The listing builds one solid part. Answer for the finished solid, in the listing's coordinates (mm). A direction names the side the tool comes from. Coordinates: 2 decimals unless noted, no trailing zeros. Order: outer loops, then holes, each group sorted by start corner. A loop starts at its lowest first (then second) coordinate and runs counter-clockwise, first axis right, second up. Notation, with made-up numbers: (3, 57.5) -> (16, 57.5) arc R14 cw to (16, 84.5) -> close; hole circle Ø2 at (-37.75, -33.5). An arc over 180 degrees is marked (long way). Write item = value, one per line.
from build123d import *
from build123d.topology import SkipClean

# Parameters (mm, degrees)
SALIENTE_EXTRUIR1_DEPTH    = 2.4
CORTAR_EXTRUIR1_DEPTH      = 43.673293756
CORTAR_EXTRUIR1_DEPTH_BACK = 43.673293756
CROQUIS2_R                 = 1.5
CROQUIS3_R                 = 1.5
SALIENTE_EXTRUIR2_DEPTH    = 7.5
CORTAR_EXTRUIR2_DEPTH      = 3.1
REDONDEO1_R                = 2
REDONDEO2_R                = 1


with BuildPart() as part:
    # Croquis1 → Saliente-Extruir1 (new, symmetric)
    with BuildSketch(Plane(origin=(0, 0, 0), x_dir=(0, 0, -1), z_dir=(1, 0, 0))):
        with BuildLine():
            Line((-41.5, 3), (41.5, 3))
            ThreePointArc((41.5, 3), (42.207106781, 2.707106781), (42.5, 2))
            Line((42.5, 2), (42.5, -2))
            ThreePointArc((42.5, -2), (42.207106781, -2.707106781), (41.5, -3))
            Line((41.5, -3), (-41.5, -3))
            ThreePointArc((-41.5, -3), (-42.207106781, -2.707106781), (-42.5, -2))
            Line((-42.5, -2), (-42.5, 2))
            ThreePointArc((-42.5, 2), (-42.207106781, 2.707106781), (-41.5, 3))
        make_face()
    extrude(amount=SALIENTE_EXTRUIR1_DEPTH, both=True)

    # Croquis2 → Cortar-Extruir1 (cut, two sides: drawn at the far end of the back side and taken through both)
    with BuildSketch(Plane(origin=(0, 0, 0), x_dir=(0, 0, -1), z_dir=(1, 0, 0)).offset(-CORTAR_EXTRUIR1_DEPTH_BACK)):
        with Locations((-38.5, 0)):
            Circle(CROQUIS2_R)
        with Locations((33.5, 0)):
            Circle(CROQUIS2_R)
    extrude(amount=CORTAR_EXTRUIR1_DEPTH + CORTAR_EXTRUIR1_DEPTH_BACK, mode=Mode.SUBTRACT)

    # Croquis3 → Saliente-Extruir2 (add, symmetric)
    with SkipClean():  # the faces are left unmerged after this step: merging them gives an invalid solid
        with BuildSketch(Plane(origin=(0, 0, 0), x_dir=(0, 0, -1), z_dir=(1, 0, 0))):
            with BuildLine():
                Line((-42.5, 2), (-42.5, -2))
                ThreePointArc((-42.5, -2), (-42.207106781, -2.707106781), (-41.5, -3))
                Line((-41.5, -3), (-27.5, -3))
                Line((-27.5, -3), (-27.5, 3))
                Line((-27.5, 3), (-41.5, 3))
                ThreePointArc((-41.5, 3), (-42.207106781, 2.707106781), (-42.5, 2))
            make_face()
            with Locations((-38.5, 0)):
                Circle(CROQUIS3_R, mode=Mode.SUBTRACT)
        extrude(amount=SALIENTE_EXTRUIR2_DEPTH, both=True)
    add(part.part.scale(1), mode=Mode.REPLACE)  # the faces are merged on a copy

    # Croquis4 → Cortar-Extruir2 (cut, symmetric)
    with BuildSketch(Plane(origin=(0, 0, 0), x_dir=(0, 0, -1), z_dir=(1, 0, 0))):
        with BuildLine():
            Line((-41.5, 3), (-32.5, 3))
            Line((-32.5, 3), (-32.5, -3))
            Line((-32.5, -3), (-41.5, -3))
            ThreePointArc((-41.5, -3), (-42.207106781, -2.707106781), (-42.5, -2))
            Line((-42.5, -2), (-42.5, 2))
            ThreePointArc((-42.5, 2), (-42.207106781, 2.707106781), (-41.5, 3))
        make_face()
    extrude(amount=CORTAR_EXTRUIR2_DEPTH, both=True, mode=Mode.SUBTRACT)

    # Redondeo1
    redondeo1_edges = [part.edges().sort_by_distance(p)[0] for p in [
        (-2.4, 0, 27.5),
        (2.4, 0, 27.5),
        (-7.5, 0, 27.5),
        (7.5, 0, 27.5),
    ]]
    fillet(redondeo1_edges, radius=REDONDEO1_R)

    # Redondeo2
    redondeo2_edges = [part.edges().sort_by_distance(p)[0] for p in [
        (3.1, 0, 32.5),
        (-3.1, 0, 32.5),
    ]]
    fillet(redondeo2_edges, radius=REDONDEO2_R)


solid = part.part
Q1. Each of these flat-tipped pins is pushed along its axis until it touches: pin 1 Ø1.5 at (y, z) = (-0.5, 8) entering from +X; pin 2 Ø1 at (y, z) = (-1, -34) entering from -X; pin 3 Ø2 at (x, y) = (-1.5, 0.5) entering from +Z. Where does it stop, or does it pass through?
The answers:
pin_1 = 2.4
pin_2 = -2.4
pin_3 = 32.58
Q2. Section A-A, the plane x = 0.5 is taken. Give the vertices of the cut face in (y, z).
The answers:
outline = (-3, -41.5) arc R1 ccw to (-2, -42.5) -> (2, -42.5) arc R1 ccw to (3, -41.5) -> (3, 32.5) -> (-3, 32.5) -> close; hole circle Ø3 at (0, -33.5)
Q3. Section D-D, the plane z = 22 is taken. Give the vertices of the cut face in (x, y), plus the area to 3 significant figures.
The answers:
outline = (-2.4, -3) -> (2.4, -3) -> (2.4, 3) -> (-2.4, 3) -> close
area = 28.8 mm2
Q4. Section B-B, the plane y = 0 is taken. Give the number of separate pieces and of enclosed holes in the cut face, plus the area to 3 significant figures.
The answers:
separate_pieces = 4
enclosed_holes = 0
area = 459 mm2
Q5. The mould has two halves that part along Y. Classify faces 4 (the face through (0, 3, -1)), 5 (the face through (0, -0.9, -32.3)), 6 (the face through (-2.4, 0, -9)): released by +Y, released by -Y, zero draft, split by the parting line, or undercut.
The answers:
face_4 = released by +Y
face_5 = undercut
face_6 = zero draft
Q6. Section C-C, the plane z = -33.5 is taken. Give the vertices of the cut face in (x, y), plus the area to 3 significant figures.
The answers:
outline = (-2.4, -3) -> (2.4, -3) -> (2.4, -1.5) -> (-2.4, -1.5) -> close; (-2.4, 1.5) -> (2.4, 1.5) -> (2.4, 3) -> (-2.4, 3) -> close
area = 14.4 mm2
Q7. Find the intervals of material crossed by line 1 along Y through (x, z) = (-5.25, 38.5); line 2 along X through (y, z) = (-0.5, -6.5); line 3 along Z through (x, y) = (-0.4, 0), in increasing order.
The answers:
line_1 = -3 to -1.5, 1.5 to 3
line_2 = -2.4 to 2.4
line_3 = -42.5 to -35, -32 to 32.5
Q8. A tool of negligible diameter and unlimited length cuts with its end or side. For faces 1 (the face through (-5.3, -0.9, 39.7)), 2 (the face through (0, 0, 32.5)), 3 (the face through (2.4, 0, -9)), from which of +Z, -Z, +X, -X, +Y, -Y can it reach the whole face along a straight path? Write none if from no direction.
The answers:
face_1 = +X, -X
face_2 = +Z, +Y, -Y
face_3 = -Z, +X, +Y, -Y
